from build123d import *

# Parameters (mm, degrees)
SKETCH2_R               = 50
BOSS_EXTRUDE1_DEPTH     = 10
SKETCH3_W               = 50
SKETCH3_H               = 50
BOSS_EXTRUDE2_DEPTH     = 60
CUT_EXTRUDE1_DEPTH      = 115.127122105
CUT_EXTRUDE2_DEPTH      = 109.12145948
CUT_EXTRUDE2_DEPTH_BACK = 109.12145948
SKETCH5_R               = 5
FILLET1_R               = 25


with BuildPart() as part:
    # Sketch2 → Boss-Extrude1 (new body)
    with BuildSketch(Plane(origin=(0, 0, 0), x_dir=(1, 0, 0), z_dir=(0, 1, 0))):
        with Locations(Location((0, 0, 0), (0, 0, 270))):
            Circle(SKETCH2_R)
    extrude(amount=BOSS_EXTRUDE1_DEPTH)

    # Sketch3 → Boss-Extrude2 (add)
    with BuildSketch(Plane(origin=(0, 10, 0), x_dir=(1, 0, 0), z_dir=(0, 1, 0))):
        Rectangle(SKETCH3_W, SKETCH3_H)
    extrude(amount=BOSS_EXTRUDE2_DEPTH)

    # Sketch4 → Cut-Extrude1 (cut, through all)
    with BuildSketch(Plane(origin=(25, 0, 0), x_dir=(0, 0, -1), z_dir=(1, 0, 0))):
        with BuildLine():
            Line((-15.5, 70), (15.5, 70))
            Line((15.5, 70), (15.5, 50))
            ThreePointArc((15.5, 50), (0, 29.724643504), (-15.5, 50))
            Line((-15.5, 50), (-15.5, 70))
        make_face()
    extrude(amount=-CUT_EXTRUDE1_DEPTH, mode=Mode.SUBTRACT)

    # Sketch5 → Cut-Extrude2 (cut, two sides: drawn at the far end of the back side and taken through both)
    with BuildSketch(Plane.XY.offset(-15.5).offset(-CUT_EXTRUDE2_DEPTH_BACK)):
        with Locations((0, 60)):
            Circle(SKETCH5_R)
    extrude(amount=CUT_EXTRUDE2_DEPTH + CUT_EXTRUDE2_DEPTH_BACK, mode=Mode.SUBTRACT)

    # Fillet1
    fillet1_edges = [part.edges().sort_by_distance(p)[0] for p in [
        (25, 70, 20.25),
        (-25, 70, 20.25),
        (-25, 70, -20.25),
        (25, 70, -20.25),
    ]]
    fillet(fillet1_edges, radius=FILLET1_R - 0.0001)  # a hair under: the kernel refuses the full size


solid = part.part
Check sheet for the modelled part. Datum: model origin and axes. Units: mm. A direction names the side the tool comes from. Round coordinates to 2 decimals unless told otherwise and drop trailing zeros. Loops run counter-clockwise (first coordinate to the right, second up) from the corner with the lowest first, then second, coordinate; pieces in that order, holes last. Notation, with made-up numbers: M -11.5,-24 L -2.5,-24 A30 cw -2.5,9 Z; hole C 21.5,7 d1. An arc over 180 degrees is marked long. One line per question, with ' | ' between items. Start each with the question number.
Item 1: Release check for a two-part mould opening along Y. For faces 1 (the face through (0.35, 29.73, -0.41)), 2 (the face through (-17.871, 62.482, -20.316)), 3 (the face through (15.02, 4.93, 47.69)) record: released by +Y, released by -Y, zero draft, split by the parting line, or undercut.
Item 2: Section check A-A (z = 0). Record the boundary of the cut face in (x, y).
Item 3: Section check D-D (y = 60). Record the boundary of the cut face in (x, z), and give its area (3 significant figures).
Item 4: Set-up check for faces 4 (the face through (1, 10, 33)), 5 (the face through (0, 53, -15.5)), 6 (the face through (-25, 23, 0)), 7 (the face through (0, 40, -25)): record each of +Z, -Z, +X, -X, +Y, -Y from which the full face is reachable in a straight line by a thin tool's end or side.
Item 5: Section check B-B (y = 52). Record the boundary of the cut face in (x, z), and give its area (3 significant figures).
Item 6: Section check C-C (x = -3). Record the boundary of the cut face in (y, z), and give its area (3 significant figures).
Item 7: Gauge pin test, flat ends, axial feed: pin 1 Ø2 at (x, y) = (10.5, 18.5) entering from -Z; pin 2 Ø8 at (x, y) = (0, 60) entering from -Z; pin 3 Ø25 at (x, y) = (-12.5, 33.5) entering from +Z; pin 4 Ø5 at (y, z) = (56.5, 25) entering from -X. Record the tip position at first contact, or that the pin passes through.
Item 8: Scan lines: probe 1 along Y at (x, z) = (0, 21); probe 2 along Z at (x, y) = (19.5, 58); probe 3 along Y at (x, z) = (-18, -30.5). Record each from-to range of solid material in increasing order.
Worked out:
1) face 1: undercut | face 2: released by +Y | face 3: zero draft
2) outline: M -50,0 L 50,0 L 50,10 L 25,10 L 25,29.72 L -25,29.72 L -25,10 L -50,10 Z
3) outline: M -20,-25 L -5,-25 L -5,-15.5 L -20,-15.5 Z; M -20,15.5 L -5,15.5 L -5,25 L -20,25 Z; M 5,-25 L 20,-25 L 20,-15.5 L 5,-15.5 Z; M 5,15.5 L 20,15.5 L 20,25 L 5,25 Z | area: 570 mm^2
4) face 4: +Y | face 5: +X, -X, +Y | face 6: +Z, -Z, -X, +Y | face 7: -Z, +X, -X, +Y
5) outline: M -24,-25 L 24,-25 L 24,-15.5 L -24,-15.5 Z; M -24,15.5 L 24,15.5 L 24,25 L -24,25 Z | area: 912 mm^2
6) outline: M 0,-49.91 L 10,-49.91 L 10,-25 L 56,-25 L 56,-15.5 L 50,-15.5 A16.06 cw long 50,15.5 L 56,15.5 L 56,25 L 10,25 L 10,49.91 L 0,49.91 Z; M 64,-25 L 69.82,-25 L 69.82,-15.5 L 64,-15.5 Z; M 64,15.5 L 69.82,15.5 L 69.82,25 L 64,25 Z | area: 2,680 mm^2
7) pin 1: z = -25 | pin 2: through | pin 3: z = 25 | pin 4: x = -23.32
8) probe 1: 0 to 55, 65 to 70 | probe 2: -25 to -15.5, 15.5 to 25 | probe 3: 0 to 10
